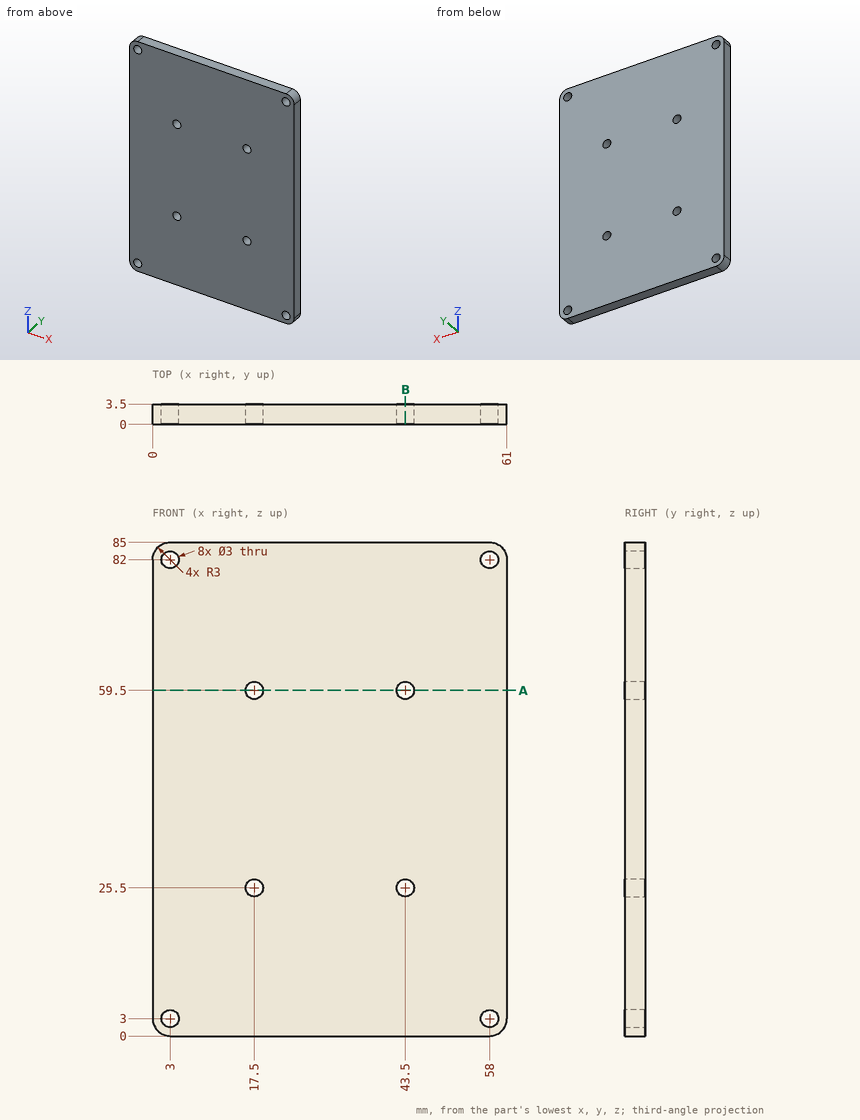
Verification items for this drawing (mm, ordinates from the low corner). Round coordinates to 2 decimals unless told otherwise and drop trailing zeros. Order: outer loops, then holes, each group sorted by start corner. A loop starts at its lowest first (then second) coordinate and runs counter-clockwise, first axis right, second up. Notation, with made-up numbers: (74.5, -14) - (128.5, -14) arc R16 ccw to (128.5, 0) - close; hole circle Ø1 at (16.25, 48). An arc over 180 degrees is marked (long way). Use CSV: the item, a comma, the result in double quotes. Start each with the question number.
1) Thickness scan on L1, parallel to X at y = 2.1, z = 3; L2, parallel to X at y = 2.3, z = 59.5; L3, parallel to Z at x = 17, y = 3. Record the ranges inside material, lowest first.
2) Go/stop test with a flat-tipped pin: P1, Ø5, axis at x = 43.5, z = 59.5, coming from the -Y side. Record where the tip stops, or that it passes through.
3) Section check B-B, the plane x = 43.5. Record the cut outline in (y, z), plus the area to 4 significant figures.
4) Section check A-A, the plane z = 59.5. Record the cut outline in (x, y), plus the area to 4 significant figures.
Answers:
1,L1,"x = 0 to 1.5, 4.5 to 56.5, 59.5 to 61"
1,L2,"x = 0 to 16, 19 to 42, 45 to 61"
1,L3,"z = 0 to 24.09, 26.91 to 58.09, 60.91 to 85"
2,P1,"stops at y = 0"
3,outline,"(0, 0) - (3.5, 0) - (3.5, 24) - (0, 24) - close; (0, 27) - (3.5, 27) - (3.5, 58) - (0, 58) - close; (0, 61) - (3.5, 61) - (3.5, 85) - (0, 85) - close"
3,area,"276.5 mm²"
4,outline,"(0, 0) - (16, 0) - (16, 3.5) - (0, 3.5) - close; (19, 0) - (42, 0) - (42, 3.5) - (19, 3.5) - close; (45, 0) - (61, 0) - (61, 3.5) - (45, 3.5) - close"
4,area,"192.5 mm²"
